Autodesk Inventor part; units mm, degrees
ref_plane "YZ Plane" through (0, 0, 0) normal (1, 0, 0) x (0, 1, 0)
ref_plane "XZ Plane" through (0, 0, 0) normal (0, 1, 0) x (-1, 0, 0)
ref_plane "XY Plane" through (0, 0, 0) normal (0, 0, 1) x (1, 0, 0)
sketch "スケッチ1" plane through (0, 0, 0) normal (0, 0, 1) x (1, 0, 0)
  circle A0 centre (0, 0) radius 17.5
  line L0 (0, 0) -> (35, 0)
  line L1 (35, 0) -> (35, 20)
  line L2 (35, 20) -> (-1.2255, 17.457)
  line L3 (35, 20) -> (85, 20)
  line L4 (85, 20) -> (85, 0)
  line L5 (85, 0) -> (35, 0)
  line L6 (35, 0) -> (35, 20)
  line L7 (35, 0) -> (35, -20)
  line L8 (35, -20) -> (-1.2255, -17.457)
  line L9 (35, -20) -> (85, -20)
  line L10 (85, -20) -> (85, 0)
  point P0 (-1.2255, -17.457)
  dimension "d0" = 35
  dimension "d1" = 35
  dimension "d2" = 20
  dimension "d3" = 20
  dimension "d4" = 50
extrude "プレート1" add sketch "スケッチ1" along normal blind 2
sketch "スケッチ2" plane through (85, 22, -2) normal (0, 1, 0) x (-1, 0, 0)
  line L0 (50, 0) -> (0, 0)
  line L1 (0, 0) -> (0, -29.5)
  line L2 (0, -29.5) -> (50, -29.5)
  line L3 (50, -29.5) -> (50, 0)
edge flange "フランジ1" height 33.5 angle 90 thickness 2 bend radius 2 thickness toward (0, 1, 0) relief tear relief width 2 relief depth 1 corner gap 2 corner form 0 edges at (60, 20, 0) (60, -20, 0) wall of the first edge with corners at (35, 22, -2) (85, 22, -2) (85, 22, -31.5) (35, 22, -31.5)
bend "曲げ1"
corner "コーナー1"
sketch "スケッチ3" plane through (0, 0, 2) normal (0, 0, 1) x (1, 0, 0)
  circle A0 centre (0, 0) radius 12
  point P0 (0, 12)
  point P1 (-10.3923, 6)
  point P2 (-10.3923, -6)
  point P3 (0, -12)
  point P4 (10.3923, -6)
  point P5 (10.3923, 6)
  dimension "d16" = 24
  dimension "d19" = 360
hole "穴1" [suppressed]
sketch "スケッチ4" plane through (0, 0, 2) normal (0, 0, 1) x (1, 0, 0)
  arc A0 (-1.2255, 17.457) -> (-1.2255, -17.457) centre (0, 0) ccw
  circle A1 centre (0, 0) radius 6.25
  dimension "d28" = 12.5
extrude "押し出し1" [suppressed]
sketch "スケッチ5" plane through (35, 24, -31.5) normal (0, 1, 0) x (1, 0, 0)
  line L0 (0, 0) -> (0, -29.5)
  line L1 (0, -10) -> (50, -10)
  line L2 (50, -29.5) -> (50, 0)
  line L3 (50, 0) -> (0, 0)
  line L4 (10, 0) -> (10, -29.5)
  line L5 (0, -29.5) -> (50, -29.5)
  point P0 (-35, -31.5)
  point P1 (20, -10)
  point P2 (40, -10)
  dimension "d31" = 10
  dimension "d32" = 10
  dimension "d33" = 10
  dimension "d34" = 20
hole "穴2" at (55, 24, -21.5) at (75, 24, -21.5) direction (0, -1, 0) diameter 3.2 end through all
sketch "スケッチ6" plane through (0, 0, 2) normal (0, 0, 1) x (1, 0, 0)
  point P0 (0, 0)
  point P1 (0, 0)
hole "穴3" at (0, 0, 2) direction (0, 0, -1) diameter 3.1 end through all
equation "\"d26\" = Thickness"
equation "\"d47\" = Thickness"
equation "\"d5\" = Thickness"
equation "\"d6\" = BendReliefWidth"
equation "\"d7\" = BendReliefDepth"
equation "\"d8\" = MinimumRemnant"
equation "\"d9\" = TransitionRadius"
equation "\"d12\" = BendRadius"
equation "\"d13\" = CornerReliefSize"
equation "\"d14\" = GapSize"
equation "\"d15\" = JacobiRadiusSize"
equation "\"BendRadius\" = Thickness"
equation "\"BendReliefWidth\" = Thickness"
equation "\"BendReliefDepth\" = 0.5 * Thickness"
equation "\"CornerReliefSize\" = 4 * Thickness"
equation "\"MinimumRemnant\" = 2 * Thickness"
equation "\"TransitionRadius\" = BendRadius"
equation "\"JacobiRadiusSize\" = BendRadius"
equation "\"GapSize\" = Thickness"
properties part number "servoplate2_forR0" material "アルミニウム 6061"
Geometry: final body of the model. Coordinates: model frame, mm. A direction names the side the tool comes from. Coordinates: 2 decimals unless noted, no trailing zeros. Order: outer loops, then holes, each group sorted by start corner. A loop starts at its lowest first (then second) coordinate and runs counter-clockwise, first axis right, second up. Notation, with made-up numbers: (0, 42) -> (22, 42) arc R31 cw to (22, 70) -> close; hole circle Ø4 at (52.25, -9). An arc over 180 degrees is marked (long way). Use CSV: the item, a comma, the result in double quotes.
1) Section A-A on y = 0. Output: boundary loops of the cut face in (x, z), then the cut area to 3 significant figures.
Findings:
outline,"(-17.5, 0) -> (-1.55, 0) -> (-1.55, 2) -> (-17.5, 2) -> close; (1.55, 0) -> (85, 0) -> (85, 2) -> (1.55, 2) -> close"
area,"199 mm^2"
2) Section D-D on z = -21.5. Output: boundary loops of the cut face in (x, y), then the cut area to 3 significant figures.
Findings:
outline,"(35, -24) -> (53.4, -24) -> (53.4, -22) -> (35, -22) -> close; (35, 22) -> (53.4, 22) -> (53.4, 24) -> (35, 24) -> close; (56.6, -24) -> (73.4, -24) -> (73.4, -22) -> (56.6, -22) -> close; (56.6, 22) -> (73.4, 22) -> (73.4, 24) -> (56.6, 24) -> close; (76.6, -24) -> (85, -24) -> (85, -22) -> (76.6, -22) -> close; (76.6, 22) -> (85, 22) -> (85, 24) -> (76.6, 24) -> close"
area,"174 mm^2"
3) Section B-B on z = -7. Output: boundary loops of the cut face in (x, y).
Findings:
outline,"(35, -24) -> (85, -24) -> (85, -22) -> (35, -22) -> close; (35, 22) -> (85, 22) -> (85, 24) -> (35, 24) -> close"
4) Pin query (flat end, axial travel): pin 1 Ø3 at (y, z) = (21.5, -15) entering from -X; pin 2 Ø4 at (x, z) = (29.5, -1.5) entering from -Y; pin 3 Ø20 at (x, y) = (44, -5.5) entering from -Z. Return the tip coordinate at first contact, or that it passes through.
Findings:
pin 1,"stops at x = 35"
pin 2,"stops at y = -19.71"
pin 3,"stops at z = 0"
5) Section C-C on x = 55. Output: boundary loops of the cut face in (y, z), then the cut area to 3 significant figures.
Findings:
outline,"(-24, -31.5) -> (-22, -31.5) -> (-22, -23.1) -> (-24, -23.1) -> close; (-24, -19.9) -> (-22, -19.9) -> (-22, -2) arc R2 cw to (-20, 0) -> (20, 0) arc R2 cw to (22, -2) -> (22, -19.9) -> (24, -19.9) -> (24, -2) arc R4 ccw to (20, 2) -> (-20, 2) arc R4 ccw to (-24, -2) -> close; (22, -31.5) -> (24, -31.5) -> (24, -23.1) -> (22, -23.1) -> close"
area,"204 mm^2"
6) Access query for faces 4 (the cylindrical face through (56.42, -23.01, -20.76)), 5 (the flat face through (60, -22, -17)). Directions: +Z, -Z, +X, -X, +Y, -Y. A direction counts if a zero-diameter tool reaches every point of the face in a straight line with its end or side. Return the directions, or none.
Findings:
face 4,"+Y, -Y"
face 5,"-Z, +X, -X"
7) Mould query, pull axis Y, two halves, no side actions, for faces 1 (the flat face through (60, -24, -17)), 2 (the flat face through (17.141, 18.746, 0.986)), 3 (the cylindrical face through (60.35, 21.43, -0.6)). Classes: +Y half, -Y half, draft (parallel to the pull), parting line (faces both ways), or undercut.
Findings:
face 1,"-Y half"
face 2,"+Y half"
face 3,"undercut"
8) Line query: line 1 (X direction, y = 22.8, z = -21.5); line 2 (Y direction, x = 72.5, z = -21.5); line 3 (X direction, y = 0, z = 1). Output: solid intervals per line, ascending.
Findings:
line 1,"x = 35 to 53.4, 56.6 to 73.4, 76.6 to 85"
line 2,"y = -24 to -22, 22 to 24"
line 3,"x = -17.5 to -1.55, 1.55 to 85"
